Verification items for this drawing (mm, ordinates from the low corner). Coordinates: 2 decimals unless noted, no trailing zeros. Order: outer loops, then holes, each group sorted by start corner. A loop starts at its lowest first (then second) coordinate and runs counter-clockwise, first axis right, second up. Notation, with made-up numbers: M 20,-4.5 L 60,-4.5 A21 ccw 60,25.5 Z; hole C 30.25,-20 d1. An arc over 180 degrees is marked long. Return JSON: item names as keys, results as strings. Group by question number.
1. Section check A-A, the plane z = 65. Record the cut outline in (x, y).
2. Section check B-B, the plane y = 2.1. Give the number of separate pieces and of enclosed holes in the cut face, plus the area to 3 significant figures.
3. Gauge pin test, flat ends, axial feed: pin 1 (0.5 mm diameter, centred on y = 3.5, z = 9, fed in from -X); pin 2 (0.5 mm diameter, centred on y = 3.5, z = 59.5, fed in from +X). Record the tip position at first contact, or that the pin passes through.
4. Material ranges on line 1 along X through (y, z) = (2.7, 75); line 2 along X through (y, z) = (3.75, 7.5); line 3 along X through (y, z) = (0.7, 4.5), recorded low to high.
5. Section check C-C, the plane z = 11. Record the cut outline in (x, y).
6. Mould release check, pull along X, two halves, no side actions. Record for the marked faces 1 and 2: +X half, -X half, draft (parallel to the pull), parting line (faces both ways), or undercut.
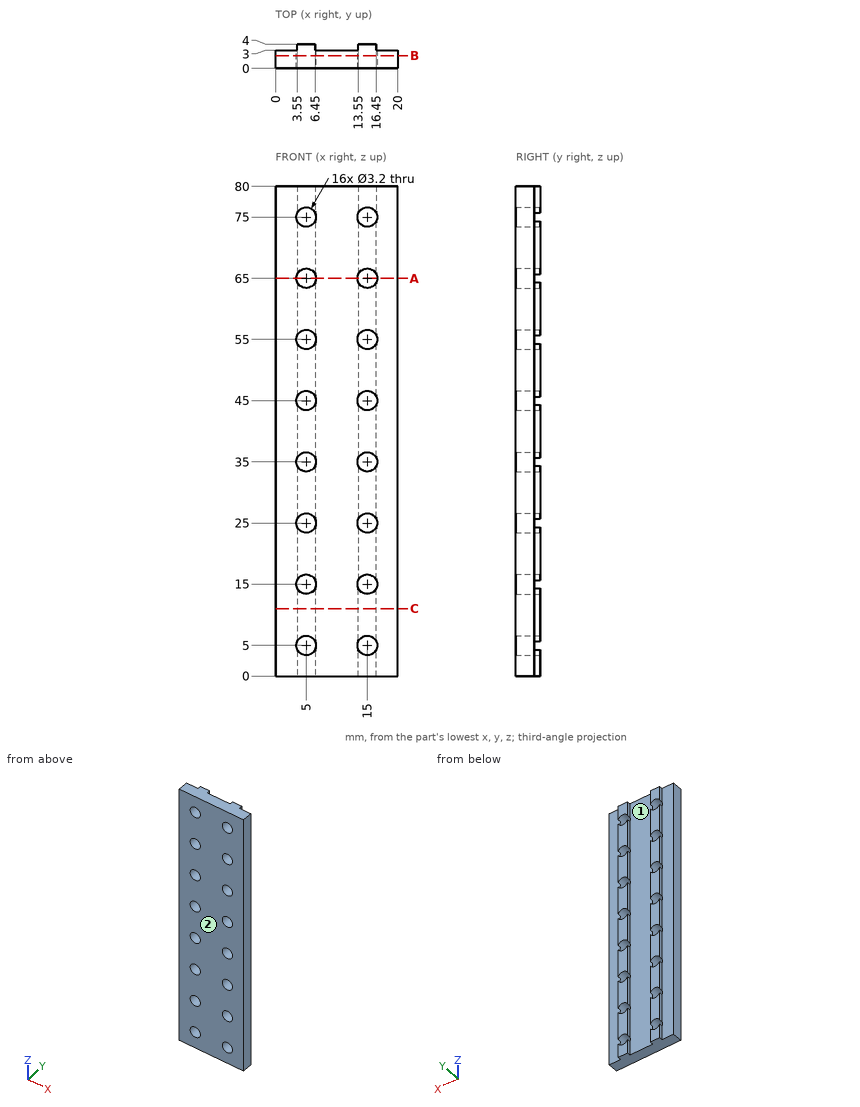
Answers follow:
{
 "1": {"outline": "M 0,0 L 3.4,0 L 3.4,3 L 0,3 Z; M 6.6,0 L 13.4,0 L 13.4,3 L 6.6,3 Z; M 16.6,0 L 20,0 L 20,3 L 16.6,3 Z"},
 "2": {"separate pieces": "1", "enclosed holes": "16", "area": "1,470 mm^2"},
 "3": {"pin 1": "x = 3.55", "pin 2": "x = 16.45"},
 "4": {"line 1": "0 to 3.4, 6.6 to 13.4, 16.6 to 20", "line 2": "3.55 to 6.45, 13.55 to 16.45", "line 3": "0 to 3.48, 6.52 to 13.48, 16.52 to 20"},
 "5": {"outline": "M 0,0 L 20,0 L 20,3 L 16.45,3 L 16.45,4 L 13.55,4 L 13.55,3 L 6.45,3 L 6.45,4 L 3.55,4 L 3.55,3 L 0,3 Z"},
 "6": {"face 1": "undercut", "face 2": "draft"}
}
